Input: part model. Units: mm. Frame: model coordinates. Round coordinates to 2 decimals unless told otherwise and drop trailing zeros. Loops run counter-clockwise (first coordinate to the right, second up) from the corner with the lowest first, then second, coordinate; pieces in that order, holes last. Notation, with made-up numbers: (-4.5, 50.25) - (31.5, 50.25) arc R9 cw to (31.5, 60.25) - close; hole circle Ø1 at (84, 53.25). An arc over 180 degrees is marked (long way). Write each question's results on one line, items separated by ' | '.
from build123d import *

# Parameters (mm, degrees)
BOSS_EXTRUDE1_DEPTH = 9
SKETCH2_W           = 14
SKETCH2_H           = 1225
CUT_EXTRUDE1_DEPTH  = 10
SKETCH3_W           = 82
SKETCH3_H           = 82
CUT_EXTRUDE2_DEPTH  = 10


with BuildPart() as part:
    # Sketch1 → Boss-Extrude1 (new body)
    with BuildSketch(Plane(origin=(0, 0, 0), x_dir=(1, 0, 0), z_dir=(0, 1, 0))):
        Polygon((-304.5, -532.5), (-304.5, -612.5), (224.5, -612.5), (304.5, -612.5), (304.5, -532.5), (304.5, 497.5), (304.5, 612.5), (224.5, 612.5), (-304.5, 612.5), (-304.5, 497.5), align=None)
    extrude(amount=BOSS_EXTRUDE1_DEPTH)

    # Sketch2 → Cut-Extrude1 (cut)
    with BuildSketch(Plane(origin=(0, 9, 0), x_dir=(1, 0, 0), z_dir=(0, 1, 0))):
        with Locations((-297.5, 0)):
            Rectangle(SKETCH2_W, SKETCH2_H)
    extrude(amount=-CUT_EXTRUDE1_DEPTH, mode=Mode.SUBTRACT)

    # Sketch3 → Cut-Extrude2 (cut)
    with BuildSketch(Plane(origin=(0, 9, 0), x_dir=(1, 0, 0), z_dir=(0, 1, 0))):
        with Locations((263.5, -571.5)):
            Rectangle(SKETCH3_W, SKETCH3_H)
        Polygon((304.5, 533), (222.5, 533), (222.5, 615), (304.5, 612.5), align=None)
    extrude(amount=-CUT_EXTRUDE2_DEPTH, mode=Mode.SUBTRACT)


solid = part.part
1. Line query: line 1 (Z direction, x = 249.5, y = 5). Output: solid intervals per line, ascending. Write a range as [from, to].
Answer:
line 1: [-533, 530.5]
2. Section query A-A, the plane y = 7. Output: boundary loops of the cut face in (x, z), plus the area to 3 significant figures.
Answer:
outline: (-290.5, -612.5) - (222.5, -612.5) - (222.5, -533) - (304.5, -533) - (304.5, 530.5) - (222.5, 530.5) - (222.5, 612.5) - (-290.5, 612.5) - close | area: 716,000 mm^2
3. Contact query for flat-ended pins moving along their axis: pin 1 (5 mm diameter, centred on x = -47.5, z = -338, fed in from -Y); pin 2 (2.5 mm diameter, centred on x = 275.5, y = 2.5, fed in from +Z). Output: stop coordinate, or through.
Answer:
pin 1: y = 0 | pin 2: z = 530.5
